Geometry check sheet. Reference: the model listing, model coordinates, mm. A direction names the side the tool comes from. Coordinates: 2 decimals unless noted, no trailing zeros. Write each loop counter-clockwise with the first axis right and the second up, starting at its lowest first coordinate (ties: lowest second). Pieces come first, ordered by that corner, then holes. Notation, with made-up numbers: M 29,13.25 L 55,13.25 A8 ccw 55,19.25 Z; hole C 70,-35.5 d3. An arc over 180 degrees is marked long. Put each result on its own line as item: value. Start each with the question number.
1) Cross-section at C-C on z = -197. Record the cut outline in (x, y), plus the area to 3 significant figures.
2) Cross-section at A-A on y = 3.5. Record the cut outline in (x, z).
3) Scan lines: line 1 along X through (y, z) = (2.5, -235.5); line 2 along X through (y, z) = (3.75, -99); line 3 along Z through (x, y) = (79.5, 5). Record each from-to range of solid material in increasing order.
4) Gauge pin test, flat ends, axial feed: pin 1 (2.5 mm diameter, centred on y = 4, z = -155, fed in from +X); pin 2 (1 mm diameter, centred on y = 1.5, z = -201, fed in from +X); pin 3 (4 mm diameter, centred on y = 8, z = -166.5, fed in from +X); pin 4 (1 mm diameter, centred on x = 45.5, y = 1.5, fed in from +Z). Record the tip position at first contact, or that the pin passes through.
5) Cross-section at B-B on x = 59. Record the cut outline in (y, z).
6) Set-up check for faces 1 (the flat face through (14, 4, -155)), 2 (the flat face through (92, 4, -155)), 3 (the flat face through (54, 0, -99)): record each of +Z, -Z, +X, -X, +Y, -Y from which the full face is reachable in a straight line by a thin tool's end or side.
Autodesk Inventor part; units mm, degrees
ref_plane "YZ Plane" through (0, 0, 0) normal (1, 0, 0) x (0, 1, 0)
ref_plane "XZ Plane" through (0, 0, 0) normal (0, 1, 0) x (-1, 0, 0)
ref_plane "XY Plane" through (0, 0, 0) normal (0, 0, 1) x (1, 0, 0)
sketch "Boceto1" plane through (0, 0, 0) normal (0, 1, 0) x (-1, 0, 0)
  line L0 (0, 0) -> (-50, 0)
  line L1 (0, -84) -> (0, 0)
  line L2 (0, -84) -> (-14, -150)
  line L3 (-14, -150) -> (-14, -166)
  line L4 (-14, -166) -> (-25, -217)
  line L5 (-25, -217) -> (-37, -243)
  line L6 (-37, -243) -> (-53, -259)
  line L7 (-106, -84) -> (-106, 0)
  line L8 (-106, -84) -> (-92, -150)
  line L9 (-92, -150) -> (-92, -166)
  line L10 (-92, -166) -> (-81, -217)
  line L11 (-81, -217) -> (-69, -243)
  line L12 (-69, -243) -> (-53, -259)
  line L13 (0, 0) -> (-106, 0)
extrude "Extrusión1" add sketch "Boceto1" along normal blind 9
fillet "Empalme1" radius 50 1 edges at (92, 4.5, -166)
fillet "Empalme2" radius 50 1 edges at (14, 4.5, -166)
fillet "Empalme3" radius 50 4 edges at (25, 4.5, -217) (81, 4.5, -217) (69, 4.5, -243) (37, 4.5, -243)
equation "\"Radio_pliegue\" = Grosor"
equation "\"Anchura_desahogo_plegado\" = Grosor"
equation "\"Profundidad_desahogo_plegado\" = 0.5 * Grosor"
equation "\"Tamaño_destalonado\" = 4 * Grosor"
equation "\"Remanente_mínimo\" = 2 * Grosor"
equation "\"Radiodetransición\" = Radio_pliegue"
equation "\"Tamaño_de_radio_de_Jacobi\" = Radio_pliegue"
equation "\"TamañoSeparación\" = Grosor"
properties part number "chasis"
Answer key:
1. outline: M 20.69,0 L 85.31,0 L 85.31,9 L 20.69,9 Z
1. area: 582 mm²
2. outline: M 0,-84 L 14,-150 L 14,-160.67 A50 ccw 15.12,-171.21 L 23.84,-211.6 A50 ccw 27.31,-222.01 L 33.26,-234.9 A50 ccw 43.31,-249.31 L 53,-259 L 62.69,-249.31 A50 ccw 72.74,-234.9 L 78.69,-222.01 A50 ccw 82.16,-211.6 L 90.88,-171.21 A50 ccw 92,-160.67 L 92,-150 L 106,-84 L 106,0 L 0,0 Z
3. line 1: x = 33.54 to 72.46
3. line 2: x = 3.18 to 102.82
3. line 3: z = -220.15 to 0
4. pin 1: stops at x = 92
4. pin 2: stops at x = 84.56
4. pin 3: stops at x = 91.85
4. pin 4: stops at z = 0
5. outline: M 0,-253 L 9,-253 L 9,0 L 0,0 Z
6. face 1: -Z, -X, +Y, -Y
6. face 2: -Z, +X, +Y, -Y
6. face 3: +Z, -Z, +X, -X, -Y
